Source: CAD feature listing. Evaluate the final solid. Frame: model axes, mm. Face numbers are marked on the shaded views. A direction names the side the tool comes from. Coordinates: 2 decimals unless noted, no trailing zeros. Loops run counter-clockwise (first coordinate to the right, second up) from the corner with the lowest first, then second, coordinate; pieces in that order, holes last.
from build123d import *

# Parameters (mm, degrees)
SKETCH1_W           = 30
SKETCH1_H           = 30
BOSS_EXTRUDE1_DEPTH = 40
CUT_EXTRUDE1_REACH  = 42
SKETCH2_R           = 0.9
CUT_EXTRUDE2_REACH  = 32
SKETCH3_W           = 5
SKETCH3_H           = 25
SKETCH4_W           = 5
SKETCH4_H           = 25
CUT_EXTRUDE3_DEPTH  = 30
FILLET1_R           = 10


with BuildPart() as part:
    # Sketch1 → Boss-Extrude1 (new body)
    with BuildSketch(Plane(origin=(0, 0, 0), x_dir=(1, 0, 0), z_dir=(0, 1, 0))):
        Rectangle(SKETCH1_W, SKETCH1_H)
    extrude(amount=BOSS_EXTRUDE1_DEPTH)

    # Sketch2 → Cut-Extrude1 (cut, up to next)
    with BuildSketch(Plane(origin=(0, 40, 0), x_dir=(1, 0, 0), z_dir=(0, 1, 0)), mode=Mode.PRIVATE) as cut_extrude1_sk1:
        Circle(SKETCH2_R)
    cut_extrude1_tool1 = extrude(cut_extrude1_sk1.sketch, amount=-CUT_EXTRUDE1_REACH, mode=Mode.PRIVATE) & part.part
    add(cut_extrude1_tool1.solids().sort_by_distance((0, 40, 0))[0], mode=Mode.SUBTRACT)

    # Sketch3 → Cut-Extrude2 (cut, up to next)
    with BuildSketch(Plane(origin=(0, 0, -15), x_dir=(-1, 0, 0), z_dir=(0, 0, -1)), mode=Mode.PRIVATE) as cut_extrude2_sk1:
        with Locations((0, 12.5)):
            Rectangle(SKETCH3_W, SKETCH3_H)
    cut_extrude2_tool1 = extrude(cut_extrude2_sk1.sketch, amount=-CUT_EXTRUDE2_REACH, mode=Mode.PRIVATE) & part.part
    add(cut_extrude2_tool1.solids().sort_by_distance((0, 12.5, -15))[0], mode=Mode.SUBTRACT)

    # Sketch4 → Cut-Extrude3 (cut)
    with BuildSketch(Plane(origin=(15, 0, 0), x_dir=(0, 0, -1), z_dir=(1, 0, 0))):
        with Locations((0, 12.5)):
            Rectangle(SKETCH4_W, SKETCH4_H)
    extrude(amount=-CUT_EXTRUDE3_DEPTH, mode=Mode.SUBTRACT)

    # Fillet1
    fillet1_edges = [part.edges().sort_by_distance(p)[0] for p in [
        (2.5, 12.5, 2.5),
        (-2.5, 12.5, 2.5),
        (2.5, 12.5, -2.5),
        (-2.5, 12.5, -2.5),
    ]]
    fillet(fillet1_edges, radius=FILLET1_R)


solid = part.part
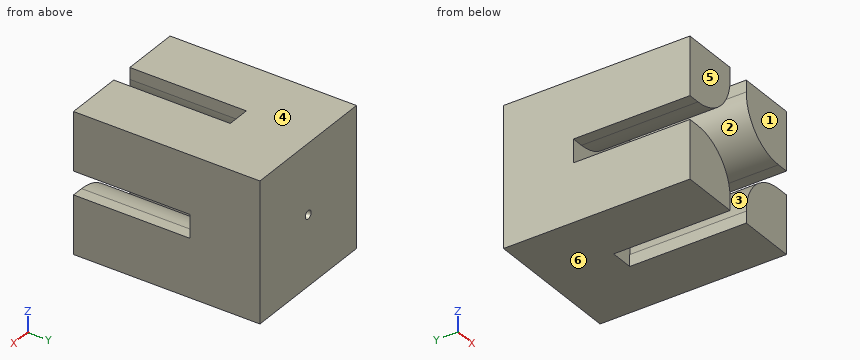
Q1. Section C-C, the plane y = 24.5. Return the cut outline in (x, z).
Q2. Line query: line 1 along X through (y, z) = (37.25, 0); line 2 along Z through (x, y) = (-13, 21.5). Output: solid intervals per line, ascending.
Q3. Section D-D, the plane z = 3. Return the cut outline in (x, y).
Q4. Section A-A, the plane z = 0. Return the cut outline in (x, y), plus the area to 3 significant figures.
Q5. Section B-B, the plane x = 0. Return the cut outline in (y, z).
Q6. Access query for the marked faces 1 and 2. Directions: +Z, -Z, +X, -X, +Y, -Y. A direction counts if a zero-diameter tool reaches every point of the face in a straight line with its end or side. Return the directions, or none.
Q7. Contact query for a flat-ended pin moving along its axis: pin 1 Ø2 at (x, z) = (0, 0) entering from -Y. Output: stop coordinate, or through.
Q8. Draft query along Z for the marked faces 3, 4, 5 and 6. Return one class per face: +Z half, -Z half, draft (parallel to the pull), parting line (faces both ways), or undercut.
Derived:
1. outline: (-15, -15) - (-2.5, -15) - (-2.5, -12.5) arc R10 ccw to (-12.5, -2.5) - (-15, -2.5) - close; (-15, 2.5) - (-12.5, 2.5) arc R10 ccw to (-2.5, 12.5) - (-2.5, 15) - (-15, 15) - close; (2.5, -15) - (15, -15) - (15, -2.5) - (12.5, -2.5) arc R10 ccw to (2.5, -12.5) - close; (2.5, 12.5) arc R10 ccw to (12.5, 2.5) - (15, 2.5) - (15, 15) - (2.5, 15) - close
2. line 1: x = -15 to -0.9, 0.9 to 15
2. line 2: z = -15 to -2.5, 2.5 to 15
3. outline: (-15, 0) - (-9.38, 0) - (-9.38, 25) - (9.38, 25) - (9.38, 0) - (15, 0) - (15, 40) - (-15, 40) - close
4. outline: (-15, 25) - (-0.9, 25) - (-0.9, 40) - (-15, 40) - close; (0.9, 25) - (15, 25) - (15, 40) - (0.9, 40) - close
4. area: 423 mm2
5. outline: (25, -15) - (40, -15) - (40, -0.9) - (25, -0.9) - close; (25, 0.9) - (40, 0.9) - (40, 15) - (25, 15) - close
6. face 1: +Z, -Z, +X, -X, -Y
6. face 2: -Y
7. pin 1: stops at y = 25
8. face 3: undercut
8. face 4: +Z half
8. face 5: draft
8. face 6: -Z half
